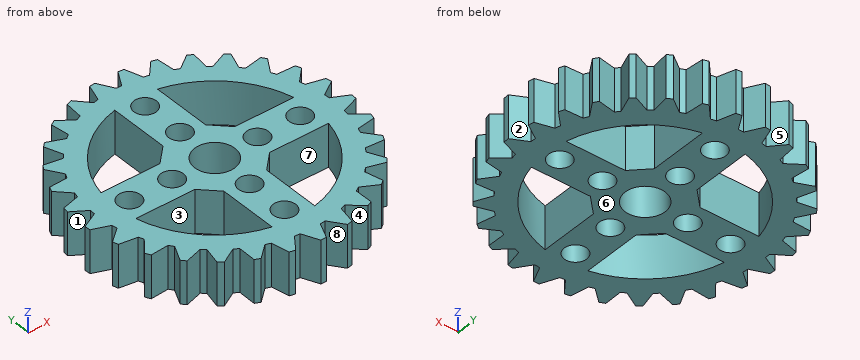
```python
from build123d import *

# Parameters (mm, degrees)
SKETCH1_R           = 25
BOSS_EXTRUDE1_DEPTH = 8
CHAMFER1_SIZE       = 3
SKETCH2_R           = 3.75
SKETCH2_R_2         = 2.1
CUT_EXTRUDE1_DEPTH  = 10
CUT_EXTRUDE4_DEPTH  = 10
CIRPATTERN1_COUNT   = 29
CIRPATTERN2_COUNT   = 4


with BuildPart() as part:
    # Sketch1 → Boss-Extrude1 (new body)
    with BuildSketch(Plane.XY):
        Circle(SKETCH1_R)
        with BuildLine():
            Line((-4, 18.062391868), (-4, 4))
            Line((-4, 4), (-18.062391868, 4))
            ThreePointArc((-18.062391868, 4), (-13.081475452, 13.081475452), (-4, 18.062391868))
        make_face(mode=Mode.SUBTRACT)
        with BuildLine():
            Line((-18.062391868, -4), (-4, -4))
            Line((-4, -4), (-4, -18.062391868))
            ThreePointArc((-4, -18.062391868), (-13.081475452, -13.081475452), (-18.062391868, -4))
        make_face(mode=Mode.SUBTRACT)
        with BuildLine():
            Line((4, -18.062391868), (4, -4))
            Line((4, -4), (18.062391868, -4))
            ThreePointArc((18.062391868, -4), (13.081475452, -13.081475452), (4, -18.062391868))
        make_face(mode=Mode.SUBTRACT)
        with BuildLine():
            Line((18.062391868, 4), (4, 4))
            Line((4, 4), (4, 18.062391868))
            ThreePointArc((4, 18.062391868), (13.081475452, 13.081475452), (18.062391868, 4))
        make_face(mode=Mode.SUBTRACT)
    extrude(amount=BOSS_EXTRUDE1_DEPTH)

    # Chamfer1
    chamfer1_edges = [part.edges().sort_by_distance(p)[0] for p in [
        (-4, 4, 4),
        (4, 4, 4),
        (-4, -4, 4),
        (4, -4, 4),
    ]]
    chamfer(chamfer1_edges, length=CHAMFER1_SIZE)

    # Sketch2 → Cut-Extrude1 (cut)
    with BuildSketch(Plane.XY.offset(8)):
        Circle(SKETCH2_R)
        with Locations((-8, 0)):
            Circle(SKETCH2_R_2)
        with Locations((-16, 0)):
            Circle(SKETCH2_R_2)
    cut_extrude1 = extrude(amount=-CUT_EXTRUDE1_DEPTH, mode=Mode.SUBTRACT)

    # Sketch3 → Cut-Extrude4 (cut)
    with BuildSketch(Plane.XY.offset(8)):
        Polygon((-2.809401077, 26), (-0.5, 22), (0.5, 22), (2.809401077, 26), align=None)
    cut_extrude4 = extrude(amount=-CUT_EXTRUDE4_DEPTH, mode=Mode.SUBTRACT)

    # CirPattern1: Cut-Extrude4 ×29 about axis
    cirpattern1_axis = Axis((0, 0, 0), (0, 0, 1))
    for i in range(1, CIRPATTERN1_COUNT):
        add(cut_extrude4.rotate(cirpattern1_axis, i * 360 / CIRPATTERN1_COUNT), mode=Mode.SUBTRACT)

    # CirPattern2: Cut-Extrude1 ×4 about axis
    cirpattern2_axis = Axis((0, 0, 0), (0, 0, 1))
    for i in range(1, CIRPATTERN2_COUNT):
        add(cut_extrude1.rotate(cirpattern2_axis, i * 360 / CIRPATTERN2_COUNT), mode=Mode.SUBTRACT)


solid = part.part
```
Source: CAD feature listing. Evaluate the final solid. Frame: model axes, mm. Face numbers are marked on the shaded views. A direction names the side the tool comes from. Give positions to 0.01 mm unless a question says otherwise; leave off trailing zeros. Loops run counter-clockwise (first coordinate to the right, second up) from the corner with the lowest first, then second, coordinate; pieces in that order, holes last. Notation, with made-up numbers: (71, 48) - (112, 48) arc R11 ccw to (112, 58) - close; hole circle Ø11 at (82.5, -15). An arc over 180 degrees is marked (long way). Use CSV: the item, a comma, the result in double quotes.
1) Pin query (flat end, axial travel): P1, Ø1.5, axis at x = -18, z = 4.5, coming from the -Y side; P2, Ø4, axis at y = -13.5, z = 2.5, coming from the +X side; P3, Ø0.8, axis at x = 0, z = 5.5, coming from the +Y side. Return the tip coordinate at first contact, or that it passes through.
Worked out:
P1,"stops at y = -16.58"
P2,"stops at x = 22.2"
P3,"stops at y = 22"
2) Cut plane B-B (z = 3.75). Count the separate pieces of the cut face and the enclosed holes in it, and give its area (3 significant figures).
Worked out:
separate pieces,"1"
enclosed holes,"13"
area,"1,040 mm^2"
3) Line query: line 1 (Y direction, x = -21.5, z = 2.25); line 2 (X direction, y = 1, z = 7); line 3 (Y direction, x = -1.5, z = 5.25). Output: solid intervals per line, ascending.
Worked out:
line 1,"y = -12.15 to -10.19, -7.55 to 5.36, 6.81 to 9.8"
line 2,"x = -21.98 to -17.85, -14.15 to -9.85, -6.15 to -3.61, 3.61 to 6.15, 9.85 to 14.15, 17.85 to 21.98"
line 3,"y = -22.79 to -17.47, -14.53 to -9.47, -6.53 to -3.44, 3.44 to 6.53, 9.47 to 14.53, 17.47 to 23.73"
4) Set-up query: the marked faces 1, 2, 3, 4 and 5. Return all of +Z, -Z, +X, -X, +Y, -Y with unobstructed straight access to the full face (end or side cutting, diameter ignored); none if empty.
Worked out:
face 1,"+Z, -Z, -X"
face 2,"+Z, -Z, +X"
face 3,"+Z, -Z"
face 4,"+Z, -Z, -Y"
face 5,"+Z, -Z, +Y"
5) Mould query, pull axis Y, two halves, no side actions, for the marked faces 6, 7 and 8. Classes: +Y half, -Y half, draft (parallel to the pull), parting line (faces both ways), or undercut.
Worked out:
face 6,"draft"
face 7,"undercut"
face 8,"-Y half"
6) Cut plane A-A (y = 0). Output: boundary loops of the cut face in (x, z), and give its area (3 significant figures).
Worked out:
outline,"(-23.36, 0) - (-18.1, 0) - (-18.1, 8) - (-23.36, 8) - close; (-13.9, 0) - (-10.1, 0) - (-10.1, 8) - (-13.9, 8) - close; (-5.9, 0) - (-3.75, 0) - (-3.75, 8) - (-5.9, 8) - close; (3.75, 0) - (5.9, 0) - (5.9, 8) - (3.75, 8) - close; (10.1, 0) - (13.9, 0) - (13.9, 8) - (10.1, 8) - close; (18.1, 0) - (23.36, 0) - (23.36, 8) - (18.1, 8) - close"
area,"179 mm^2"
7) Cut plane C-C (y = 16). Output: boundary loops of the cut face in (x, z).
Worked out:
outline,"(-16.94, 0) - (-9.29, 0) - (-9.29, 8) - (-16.94, 8) - close; (-4, 0) - (-2.1, 0) - (-2.1, 8) - (-4, 8) - close; (2.1, 0) - (4, 0) - (4, 8) - (2.1, 8) - close; (9.29, 0) - (16.94, 0) - (16.94, 8) - (9.29, 8) - close"
